CAD build for the part. Positions are in the model's coordinates, mm. Give positions to 0.01 mm unless a question says otherwise; leave off trailing zeros. Loops run counter-clockwise (first coordinate to the right, second up) from the corner with the lowest first, then second, coordinate; pieces in that order, holes last. Notation, with made-up numbers: (23.5, 51) -> (66.5, 51) arc R26 ccw to (66.5, 83) -> close; hole circle Ø9 at (51, 36.25). An arc over 180 degrees is marked (long way). Use one line per item in the form item = value.
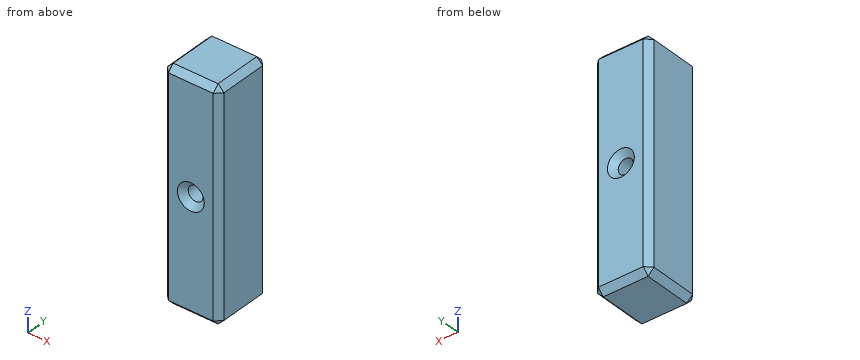
```python
from build123d import *

# Parameters (mm, degrees)
F0_W     = 9.5
F0_H     = 38
F1_DEPTH = 10
F2_R     = 1.25
F3_DEPTH = 25
F4_SIZE  = 1


with BuildPart() as f1:
    # F0 (on Front) → F1 (new body)
    with BuildSketch(Plane.XZ):
        with Locations((-21.8694014475, 16.620930075)):
            Rectangle(F0_W, F0_H)
    extrude(amount=F1_DEPTH)

    # F2 (on face) → F3 (cut)
    with BuildSketch(Plane.XZ.offset(10)):
        with Locations((-21.8694014475, 16.620930075)):
            Circle(F2_R)
    extrude(amount=-F3_DEPTH, mode=Mode.SUBTRACT)

    # F4
    f4_edges = [f1.edges().sort_by_distance(p)[0] for p in [
        (-21.869401, -10, 35.62093),
        (-17.119401, -10, 16.62093),
        (-26.619401, -10, 16.62093),
        (-21.869401, -10, -2.37907),
        (-23.119401, -10, 16.62093),
        (-21.869401, 0, 35.62093),
        (-17.119401, 0, 16.62093),
        (-26.619401, 0, 16.62093),
        (-21.869401, 0, -2.37907),
        (-23.119401, 0, 16.62093),
        (-26.619401, -5, 35.62093),
        (-26.619401, -5, -2.37907),
        (-17.119401, -5, -2.37907),
        (-17.119401, -5, 35.62093),
    ]]
    chamfer(f4_edges, length=F4_SIZE)


solid = f1.part
```
1. Cut at B-B, the plane z = 3.5. Write the cut outline in (x, y), then the cut area to 3 significant figures.
Result sheet:
outline = (-26.62, -9) -> (-25.62, -10) -> (-18.12, -10) -> (-17.12, -9) -> (-17.12, -1) -> (-18.12, 0) -> (-25.62, 0) -> (-26.62, -1) -> close
area = 93.0 mm^2
2. Cut at C-C, the plane x = -17.5. Write the cut outline in (y, z), then the cut area to 3 significant figures.
Result sheet:
outline = (-9.38, -1.38) -> (-9, -1.76) -> (-1, -1.76) -> (-0.62, -1.38) -> (-0.62, 34.62) -> (-1, 35) -> (-9, 35) -> (-9.38, 34.62) -> close
area = 322 mm^2
3. Drill centre lines: line 1 (Z direction, x = -22, y = -6.5); line 2 (X direction, y = -8.75, z = 15.5); line 3 (Z direction, x = -22.75, y = -6.25). Where is each one in solid material? Low to high.
Result sheet:
line_1 = -2.38 to 15.38, 17.86 to 35.62
line_2 = -26.62 to -22.42, -21.32 to -17.12
line_3 = -2.38 to 15.73, 17.51 to 35.62
4. Cut at A-A, the plane y = -1.75. Write the cut outline in (x, z), then the cut area to 3 significant figures.
Result sheet:
outline = (-26.62, -1.38) -> (-25.62, -2.38) -> (-18.12, -2.38) -> (-17.12, -1.38) -> (-17.12, 34.62) -> (-18.12, 35.62) -> (-25.62, 35.62) -> (-26.62, 34.62) -> close; hole circle Ø2.5 at (-21.87, 16.62)
area = 354 mm^2
5. Drop a flat-ended pin along its axis: P1, Ø2, axis at x = -21.87, z = 16.62, coming from the +Y side. Give the stop position or say it passes through.
Result sheet:
P1 = through
